```python
from build123d import *

# Parameters (mm, degrees)
ESBO_O1_R                = 21.25
RESSALTO_EXTRUS_O1_DEPTH = 24.25
ESBO_O2_R                = 2.5
RESSALTO_EXTRUS_O2_DEPTH = 19
ESBO_O3_R                = 1.5
CORTE_EXTRUS_O1_DEPTH    = 2


with BuildPart() as part:
    # Esboço1 → Ressalto-extrusão1 (new, symmetric)
    with BuildSketch(Plane.XY):
        with Locations(Location((0, 0, 0), (0, 0, 180))):
            Circle(ESBO_O1_R)
    extrude(amount=RESSALTO_EXTRUS_O1_DEPTH, both=True)

    # Esboço2 → Ressalto-extrusão2 (add)
    with BuildSketch(Plane(origin=(0, 0, -24.25), x_dir=(-1, 0, 0), z_dir=(0, 0, -1))):
        with Locations(Location((0, 0, 0), (0, 0, 180))):
            Circle(ESBO_O2_R)
    extrude(amount=RESSALTO_EXTRUS_O2_DEPTH)

    # Esboço3 → Corte-extrusão1 (cut)
    with BuildSketch(Plane(origin=(0, 0, -24.25), x_dir=(-1, 0, 0), z_dir=(0, 0, -1))):
        with Locations((-8.672819651, 9.001788672)):
            Circle(ESBO_O3_R)
        with Locations((9.001788672, 8.672819651)):
            Circle(ESBO_O3_R)
        with Locations((8.672819651, -9.001788672)):
            Circle(ESBO_O3_R)
        with Locations((-9.001788672, -8.672819651)):
            Circle(ESBO_O3_R)
    extrude(amount=-CORTE_EXTRUS_O1_DEPTH, mode=Mode.SUBTRACT)


solid = part.part
```
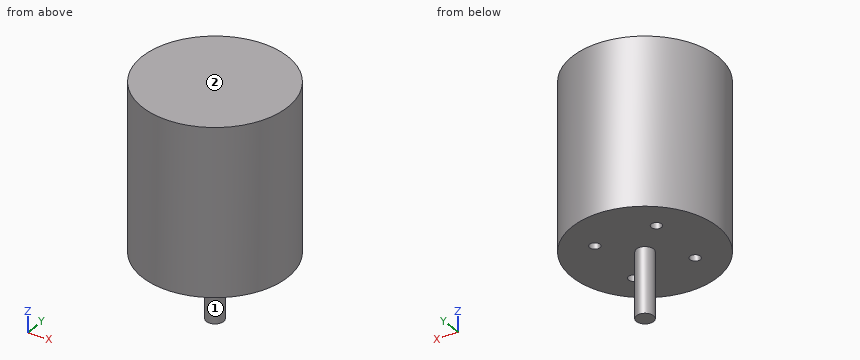
Geometry check sheet. Reference: the model listing, model coordinates, mm. Face numbers are marked on the shaded views. A direction names the side the tool comes from. Give positions to 0.01 mm unless a question says otherwise; leave off trailing zeros. Loops run counter-clockwise (first coordinate to the right, second up) from the corner with the lowest first, then second, coordinate; pieces in that order, holes last. Notation, with made-up numbers: M 50.25,64 L 94.25,64 A6 cw 94.25,70 Z; hole C 4,-23.75 d10. An arc over 180 degrees is marked long. Write item = value, one per line.
(1) Sectioned sample at C-C, the plane z = -23.5. Record the cut outline in (x, y), plus the area to 3 significant figures.
Answer below:
outline = C 0,0 d42.5; hole C -9,8.67 d3; hole C -8.67,-9 d3; hole C 8.67,9 d3; hole C 9,-8.67 d3
area = 1,390 mm2
(2) Material ranges on line 1 (Z direction, x = 8, y = 6); line 2 (Y direction, x = -19, z = 3.5); line 3 (Y direction, x = -11, z = -11), recorded low to high. Write a range as [from, to].
Answer below:
line_1 = [-24.25, 24.25]
line_2 = [-9.52, 9.52]
line_3 = [-18.18, 18.18]
(3) Sectioned sample at A-A, the plane y = 0. Record the cut outline in (x, z), plus the area to 3 significant figures.
Answer below:
outline = M -21.25,-24.25 L -2.5,-24.25 L -2.5,-43.25 L 2.5,-43.25 L 2.5,-24.25 L 21.25,-24.25 L 21.25,24.25 L -21.25,24.25 Z
area = 2,160 mm2
(4) Sectioned sample at D-D, the plane z = 7. Record the cut outline in (x, y), plus the area to 3 significant figures.
Answer below:
outline = C 0,0 d42.5
area = 1,420 mm2
(5) Tool access check on the marked faces 1 and 2. Record the directions out of +Z, -Z, +X, -X, +Y, -Y that give a thin tool (end or side, any length) a straight path to the whole face; none if there is none.
Answer below:
face_1 = -Z
face_2 = +Z, +X, -X, +Y, -Y
(6) Gauge pin test, flat ends, axial feed: pin 1 Ø3.5 at (x, y) = (8.5, 9) entering from -Z; pin 2 Ø1 at (x, z) = (6.5, -19.5) entering from -Y; pin 3 Ø0.9 at (x, y) = (8.5, -8.5) entering from -Z. Record the tip position at first contact, or that the pin passes through.
Answer below:
pin_1 = -24.25
pin_2 = -20.39
pin_3 = -22.25
